Geometry: final body of the model. Coordinates: model frame, mm. A direction names the side the tool comes from. Coordinates: 2 decimals unless noted, no trailing zeros. Write each loop counter-clockwise with the first axis right and the second up, starting at its lowest first coordinate (ties: lowest second). Pieces come first, ordered by that corner, then holes. Notation, with made-up numbers: M -14,39.25 L 8,39.25 A16 ccw 8,52.25 Z; hole C 29,-26.5 d6. An arc over 180 degrees is marked long. Write item = value, one per line. Start each with the question number.
Item 1: Pull-direction query (Y, two-part tool) for faces 3 (the flat face through (-0.07, -22.474, 22.926)), 4 (the flat face through (-5, -7, -33)), 5 (the cylindrical face through (-0.07, 3.14, -44.1)); classes: +Y half, -Y half, draft (parallel to the pull), parting line (faces both ways), or undercut.
Item 2: Reachability of faces 1 (the flat face through (-0.07, -13.755, 3.825)), 2 (the cylindrical face through (-0.07, 3.1, -25.86)) from +Z, -Z, +X, -X, +Y, -Y: full face, straight path, thin tool, end or side. Return the list, or none.
Item 3: Section B-B on x = 3. Give the number of separate pieces and of enclosed holes in the cut face, plus the area to 3 significant figures.
Item 4: First-contact query: pin 1 Ø19 at (y, z) = (0, 0) entering from +X; pin 2 Ø7 at (y, z) = (-20, 34.64) entering from +X; pin 3 Ø5 at (x, z) = (1.5, -74.5) entering from +Y; pin 4 Ø2 at (x, z) = (-0.5, -14) entering from +Y. Flat tips, straight axial feed; report the tip coordinate or a pass-through.
Item 5: Section A-A on y = -20. Output: boundary loops of the cut face in (x, z).
Item 6: Ray query, L1, parallel to Z at x = -3, y = 0; L2, parallel to Z at x = -1.75, y = -20; L3, parallel to Y at x = 4.25, z = -28.5. Return the intervals inside material, ascending. Write a range as [from, to].
Autodesk Inventor part; units mm, degrees
ref_plane "YZ Plane" through (0, 0, 0) normal (1, 0, 0) x (0, 1, 0)
ref_plane "XZ Plane" through (0, 0, 0) normal (0, 1, 0) x (-1, 0, 0)
ref_plane "XY Plane" through (0, 0, 0) normal (0, 0, 1) x (1, 0, 0)
sketch "草圖1" plane through (0, 0, 0) normal (1, 0, 0) x (0, 1, 0)
  line L0 (0, 0) -> (0, -113.9)
  line L1 (0, 0) -> (-20, 34.641016)
  circle A0 centre (0, 0) radius 6
  circle A1 centre (0, 0) radius 8
  circle A2 centre (-20, 34.641016) radius 6
  circle A3 centre (-20, 34.641016) radius 8
  circle A4 centre (0, -113.9) radius 6
  circle A5 centre (0, -113.9) radius 8
  line L2 (-13.071797, 38.641016) -> (-3.071797, 21.320508)
  line L3 (-3.071797, 21.320508) -> (2.392305, 19.856406)
  line L4 (2.392305, 19.856406) -> (14.892305, -1.794229)
  line L5 (14.892305, -1.794229) -> (7.984989, -114.389849)
  line L6 (-26.928203, 30.641016) -> (-16.928203, 13.320508)
  line L7 (-16.928203, 13.320508) -> (-17.660254, 10.588457)
  line L8 (-17.660254, 10.588457) -> (-10.160254, -2.401924)
  line L9 (-10.160254, -2.401924) -> (-7.998501, -114.054862)
  line L10 (4, -25) -> (-4, -25)
  line L11 (-4, -25) -> (-4, -45)
  line L12 (-4, -45) -> (4, -45)
  line L13 (4, -45) -> (4, -25)
  line L14 (4, -61.9) -> (-4, -61.9)
  line L15 (-4, -61.9) -> (-4, -81.9)
  line L16 (-4, -81.9) -> (4, -81.9)
  line L17 (4, -81.9) -> (4, -61.9)
  point P0 (0, -25)
  point P1 (0, -61.9)
  dimension "d0" = 113.9
  dimension "d1" = 40
  dimension "d2" = 150
  dimension "d3" = 12
  dimension "d4" = 16
  dimension "d5" = 12
  dimension "d6" = 16
  dimension "d7" = 12
  dimension "d8" = 16
  dimension "d9" = 25
  dimension "d10" = 15
  dimension "d11" = 135
  dimension "d12" = 135
  dimension "d13" = 20
  dimension "d14" = 20
  dimension "d15" = 10
  dimension "d16" = 12
  dimension "d21" = 20
  dimension "d22" = 8
  dimension "d23" = 25
  dimension "d25" = 32
sketch "草圖1 outline for 擠出1" plane through (0, 0, 0) normal (1, 0, 0) x (0, 1, 0)
  line L0 (7.984989, -114.389849) -> (14.892305, -1.794229)
  arc A0 (-7.998501, -114.054862) -> (7.984989, -114.389849) centre (0, -113.9) ccw
  line L1 (14.892305, -1.794229) -> (2.392305, 19.856406)
  line L2 (-10.160254, -2.401924) -> (-7.998501, -114.054862)
  line L3 (2.392305, 19.856406) -> (-3.071797, 21.320508)
  line L4 (-17.660254, 10.588457) -> (-10.160254, -2.401924)
  line L5 (-3.071797, 21.320508) -> (-13.071797, 38.641016)
  line L6 (-16.928203, 13.320508) -> (-17.660254, 10.588457)
  arc A1 (-13.071797, 38.641016) -> (-26.928203, 30.641016) centre (-20, 34.641016) ccw
  line L7 (-26.928203, 30.641016) -> (-16.928203, 13.320508)
  circle A2 centre (0, -113.9) radius 6
  line L8 (-4, -61.9) -> (4, -61.9)
  line L9 (-4, -81.9) -> (-4, -61.9)
  line L10 (4, -81.9) -> (-4, -81.9)
  line L11 (4, -61.9) -> (4, -81.9)
  circle A3 centre (-20, 34.641016) radius 6
  line L12 (-4, -25) -> (4, -25)
  line L13 (-4, -45) -> (-4, -25)
  line L14 (4, -45) -> (-4, -45)
  line L15 (4, -25) -> (4, -45)
  circle A4 centre (0, 0) radius 6
extrude "擠出1" add sketch "草圖1 outline for 擠出1" along normal mid plane 10
fillet "圓角2" radius 3 8 edges at (0, 4, -45) (0, 4, -25) (0, -4, -25) (0, -4, -45) (0, -4, -61.9) (0, 4, -61.9) (0, -4, -81.9) (0, 4, -81.9)
fillet "圓角3" radius 5 6 edges at (0, 14.8923, -1.7942) (0, 2.3923, 19.8564) (0, -3.0718, 21.3205) (0, -16.9282, 13.3205) (0, -17.6603, 10.5885) (0, -10.1603, -2.4019)
equation "\"d5\" = d3"
equation "\"d6\" = d4"
equation "\"d7\" = d3"
equation "\"d8\" = d4"
equation "\"d12\" = d11"
equation "\"d14\" = d13"
properties part number "Link_ECH" material "ABS 塑膠"
Responses:
q1.face_3 = -Y half
q1.face_4 = draft
q1.face_5 = undercut
q2.face_1 = -Z, +X, -X, -Y
q2.face_2 = +X, -X
q3.separate_pieces = 1
q3.enclosed_holes = 5
q3.area = 2,670 mm²
q4.pin_1 = 5
q4.pin_2 = through
q4.pin_3 = 10.59
q4.pin_4 = 14.2
q5.outline = M -5,18.64 L 5,18.64 L 5,28.64 L -5,28.64 Z; M -5,40.64 L 5,40.64 L 5,42.64 L -5,42.64 Z
q6.L1 = [-121.9, -119.9], [-107.9, -81.9], [-61.9, -45], [-25, -6], [6, 20.5]
q6.L2 = [18.64, 28.64], [40.64, 42.64]
q6.L3 = [-9.65, -4], [4, 13.25]
